Part model, mm, in its own coordinate system. A direction names the side the tool comes from. Round coordinates to 2 decimals unless told otherwise and drop trailing zeros. Write each loop counter-clockwise with the first axis right and the second up, starting at its lowest first coordinate (ties: lowest second). Pieces come first, ordered by that corner, then holes. Notation, with made-up numbers: (49, 0.25) -> (79, 0.25) arc R13 cw to (79, 11.25) -> close; hole circle Ø2 at (26, -11). An arc over 180 degrees is marked (long way). Use CSV: the item, a comma, the result in double quotes. Start each with the question number.
(1) Two-plate mould, pull along X, no slides. Class faces 1 (the flat face through (0, 12, 3.175)), 2 (the flat face through (-0.635, -9, 1)): released by +X, released by -X, zero draft, split by the parting line, or undercut.
(2) Which spindle directions (+Z, -Z, +X, -X, +Y, -Y) get a long thin tool onto all of the face, cutting with end or side? Do faces 3 (the flat face through (4.064, 0, 1)), 4 (the cylindrical face through (-4.556, -4.469, 1.436)), 5 (the cylindrical face through (10.37, -4.81, 1.89)), 6 (the cylindrical face through (8.496, -9.124, 1.61)). Say none if no direction does.
(3) Saw through at B-B (z = 1.15). Give the cut face in (x, y) (1 decimal).
(4) Saw through at A-A (x = 0). Give the cut face in (y, z) (3 decimals).
(5) Saw through at C-C (y = 1.25). Give the cut face in (x, z) (3 decimals).
(6) Saw through at D-D (x = -10.5). Give the cut face in (y, z) (3 decimals), plus the area to 4 significant figures.
(7) Drop flat-ended pins along their axis: pin 1 (1.3 mm diameter, centred on x = 8.5, z = 2, fed in from -Y); pin 2 (0.8 mm diameter, centred on y = 8.5, z = 1, fed in from -X); pin 3 (1.5 mm diameter, centred on x = -4, y = -5.5, fed in from -Z); pin 4 (5.5 mm diameter, centred on x = -4, y = -5, fed in from +Z). Give the stop position or say it passes through.
(8) Probe line 1 (X direction, y = 4, z = 2.2); line 2 (Y direction, x = 1.5, z = 1.05); line 3 (X direction, y = 5.5, z = 1.45). List the from-to ranges inside material, lowest first. Write a range as [from, to].
```python
from build123d import *

# Parameters (mm, degrees)
F0_W     = 8.128
F0_H     = 8.128
F1_DEPTH = 2.2606
F2_DEPTH = 0.635
F3_DEPTH = 3.175
F4_R     = 0.635


with BuildPart() as f1:
    # F0 (on Top) → F1 (new body)
    with BuildSketch(Plane.XY):
        with BuildLine():
            ThreePointArc((-6.3506963536, -0.635), (-4.5130128061, -4.5130128061), (-0.635, -6.3506963536))
            ThreePointArc((-0.635, -6.3506963536), (0, -6.3823639175), (0.635, -6.3506963536))
            ThreePointArc((0.635, -6.3506963536), (4.5130128061, -4.5130128061), (6.3506963536, -0.635))
            ThreePointArc((6.3506963536, -0.635), (6.3744421102, -0.3178945716), (6.3823639175, 0))
            ThreePointArc((6.3823639175, 0), (6.3744421102, 0.3178945716), (6.3506963536, 0.635))
            ThreePointArc((6.3506963536, 0.635), (4.5130128061, 4.5130128061), (0.635, 6.3506963536))
            ThreePointArc((0.635, 6.3506963536), (0, 6.3823639175), (-0.635, 6.3506963536))
            ThreePointArc((-0.635, 6.3506963536), (-4.5130128061, 4.5130128061), (-6.3506963536, 0.635))
            ThreePointArc((-6.3506963536, 0.635), (-6.3823639175, 0), (-6.3506963536, -0.635))
        make_face()
        Rectangle(F0_W, F0_H, mode=Mode.SUBTRACT)
        with BuildLine():
            Line((-0.635, -6.3506963536), (-0.635, -11.4123474798))
            ThreePointArc((-0.635, -11.4123474798), (0, -11.43), (0.635, -11.4123474798))
            Line((0.635, -11.4123474798), (0.635, -6.3506963536))
            ThreePointArc((0.635, -6.3506963536), (0, -6.3823639175), (-0.635, -6.3506963536))
        make_face()
        with BuildLine():
            ThreePointArc((0.635, 11.4123474798), (0, 11.43), (-0.635, 11.4123474798))
            Line((-0.635, 11.4123474798), (-0.635, 6.3506963536))
            ThreePointArc((-0.635, 6.3506963536), (0, 6.3823639175), (0.635, 6.3506963536))
            Line((0.635, 6.3506963536), (0.635, 11.4123474798))
        make_face()
        with BuildLine():
            Line((-8.8723474798, 0.635), (-8.8723474798, -0.635))
            Line((-8.8723474798, -0.635), (-6.3506963536, -0.635))
            ThreePointArc((-6.3506963536, -0.635), (-6.3823639175, 0), (-6.3506963536, 0.635))
            Line((-6.3506963536, 0.635), (-8.8723474798, 0.635))
        make_face()
        with BuildLine():
            Line((6.3506963536, -0.635), (8.8723474798, -0.635))
            Line((8.8723474798, -0.635), (8.8723474798, 0.635))
            Line((8.8723474798, 0.635), (6.3506963536, 0.635))
            ThreePointArc((6.3506963536, 0.635), (6.3744421102, 0.3178945716), (6.3823639175, 0))
            ThreePointArc((6.3823639175, 0), (6.3744421102, -0.3178945716), (6.3506963536, -0.635))
        make_face()
    extrude(amount=F1_DEPTH)

    # F0 (on Top) → F2 (join)
    with BuildSketch(Plane.XY):
        with BuildLine():
            ThreePointArc((-0.635, 11.4123474798), (-8.082230509, 8.082230509), (-11.4123474798, 0.635))
            Line((-11.4123474798, 0.635), (-8.8723474798, 0.635))
            Line((-8.8723474798, 0.635), (-6.3506963536, 0.635))
            ThreePointArc((-6.3506963536, 0.635), (-4.5130128061, 4.5130128061), (-0.635, 6.3506963536))
            Line((-0.635, 6.3506963536), (-0.635, 11.4123474798))
        make_face()
        with BuildLine():
            Line((8.8723474798, 0.635), (11.4123474798, 0.635))
            ThreePointArc((11.4123474798, 0.635), (8.082230509, 8.082230509), (0.635, 11.4123474798))
            Line((0.635, 11.4123474798), (0.635, 6.3506963536))
            ThreePointArc((0.635, 6.3506963536), (4.5130128061, 4.5130128061), (6.3506963536, 0.635))
            Line((6.3506963536, 0.635), (8.8723474798, 0.635))
        make_face()
        with BuildLine():
            ThreePointArc((0.635, -11.4123474798), (4.4682903074, -10.5204221269), (7.7718069116, -8.3811644375))
            ThreePointArc((7.7718069116, -8.3811644375), (10.3445014767, -4.8617064081), (11.4123474798, -0.635))
            Line((11.4123474798, -0.635), (8.8723474798, -0.635))
            Line((8.8723474798, -0.635), (6.3506963536, -0.635))
            ThreePointArc((6.3506963536, -0.635), (4.5130128061, -4.5130128061), (0.635, -6.3506963536))
            Line((0.635, -6.3506963536), (0.635, -11.4123474798))
        make_face()
        with BuildLine():
            ThreePointArc((-11.4123474798, -0.635), (-10.3445014767, -4.8617064081), (-7.7718069116, -8.3811644375))
            ThreePointArc((-7.7718069116, -8.3811644375), (-4.4682903074, -10.5204221269), (-0.635, -11.4123474798))
            Line((-0.635, -11.4123474798), (-0.635, -6.3506963536))
            ThreePointArc((-0.635, -6.3506963536), (-4.5130128061, -4.5130128061), (-6.3506963536, -0.635))
            Line((-6.3506963536, -0.635), (-8.8723474798, -0.635))
            Line((-8.8723474798, -0.635), (-11.4123474798, -0.635))
        make_face()
    extrude(amount=F2_DEPTH)

    # F0 (on Top) → F3 (join)
    with BuildSketch(Plane.XY):
        with BuildLine():
            ThreePointArc((-11.4123474798, 0.635), (-11.43, 0), (-11.4123474798, -0.635))
            Line((-11.4123474798, -0.635), (-8.8723474798, -0.635))
            Line((-8.8723474798, -0.635), (-8.8723474798, 0.635))
            Line((-8.8723474798, 0.635), (-11.4123474798, 0.635))
        make_face()
        with BuildLine():
            Line((8.8723474798, -0.635), (11.4123474798, -0.635))
            ThreePointArc((11.4123474798, -0.635), (11.4255860177, -0.317622658), (11.43, 0))
            ThreePointArc((11.43, 0), (11.4255860177, 0.317622658), (11.4123474798, 0.635))
            Line((11.4123474798, 0.635), (8.8723474798, 0.635))
            Line((8.8723474798, 0.635), (8.8723474798, -0.635))
        make_face()
        with BuildLine():
            ThreePointArc((8.4214084723, -9.5063073453), (11.581059701, -5.2123944786), (12.7, 0))
            ThreePointArc((12.7, 0), (-5.2123944786, 11.581059701), (-8.4214084723, -9.5063073453))
            Line((-8.4214084723, -9.5063073453), (-7.7718069116, -8.3811644375))
            ThreePointArc((-7.7718069116, -8.3811644375), (-10.3445014767, -4.8617064081), (-11.4123474798, -0.635))
            ThreePointArc((-11.4123474798, -0.635), (-11.43, 0), (-11.4123474798, 0.635))
            ThreePointArc((-11.4123474798, 0.635), (-8.082230509, 8.082230509), (-0.635, 11.4123474798))
            ThreePointArc((-0.635, 11.4123474798), (0, 11.43), (0.635, 11.4123474798))
            ThreePointArc((0.635, 11.4123474798), (8.082230509, 8.082230509), (11.4123474798, 0.635))
            ThreePointArc((11.4123474798, 0.635), (11.4255860177, 0.317622658), (11.43, 0))
            ThreePointArc((11.43, 0), (11.4255860177, -0.317622658), (11.4123474798, -0.635))
            ThreePointArc((11.4123474798, -0.635), (10.3445014767, -4.8617064081), (7.7718069116, -8.3811644375))
            Line((7.7718069116, -8.3811644375), (8.4214084723, -9.5063073453))
        make_face()
    extrude(amount=F3_DEPTH)

    # F4
    f4_edges = [f1.edges().sort_by_distance(p)[0] for p in [
        (-8.421408, -9.506307, 1.5875),
        (8.421408, -9.506307, 1.5875),
    ]]
    fillet(f4_edges, radius=F4_R)


solid = f1.part
```
Answers:
1,face 1,"zero draft"
1,face 2,"undercut"
2,face 3,"+Z, -Z"
2,face 4,"+Z, -Y"
2,face 5,"+Z"
2,face 6,"+Z, -Z, -Y"
3,outline,"(-11.4, -0.6) -> (-6.4, -0.6) arc R6.4 ccw to (-0.6, -6.4) -> (-0.6, -11.4) arc R11.4 ccw to (0.6, -11.4) -> (0.6, -6.4) arc R6.4 ccw to (6.4, -0.6) -> (11.4, -0.6) arc R11.4 cw to (7.8, -8.4) -> (8, -8.8) arc R0.6 ccw to (9, -8.9) arc R12.7 ccw (long way) to (-9, -8.9) arc R0.6 ccw to (-8, -8.8) -> (-7.8, -8.4) arc R11.4 cw to start; hole (-11.4, 0.6) -> (-6.4, 0.6) arc R6.4 cw to (-0.6, 6.4) -> (-0.6, 11.4) arc R11.4 ccw to start; hole (-4.1, -4.1) -> (4.1, -4.1) -> (4.1, 4.1) -> (-4.1, 4.1) -> close; hole (0.6, 6.4) arc R6.4 cw to (6.4, 0.6) -> (11.4, 0.6) arc R11.4 ccw to (0.6, 11.4) -> close"
4,outline,"(-11.43, 0) -> (-4.064, 0) -> (-4.064, 2.261) -> (-11.43, 2.261) -> close; (4.064, 0) -> (12.7, 0) -> (12.7, 3.175) -> (11.43, 3.175) -> (11.43, 2.261) -> (4.064, 2.261) -> close"
5,outline,"(-12.638, 0) -> (-4.064, 0) -> (-4.064, 2.261) -> (-6.259, 2.261) -> (-6.259, 0.635) -> (-11.361, 0.635) -> (-11.361, 3.175) -> (-12.638, 3.175) -> close; (4.064, 0) -> (12.638, 0) -> (12.638, 3.175) -> (11.361, 3.175) -> (11.361, 0.635) -> (6.259, 0.635) -> (6.259, 2.261) -> (4.064, 2.261) -> close"
6,outline,"(-7.144, 0) -> (7.144, 0) -> (7.144, 3.175) -> (4.516, 3.175) -> (4.516, 0.635) -> (0.635, 0.635) -> (0.635, 3.175) -> (-0.635, 3.175) -> (-0.635, 0.635) -> (-4.516, 0.635) -> (-4.516, 3.175) -> (-7.144, 3.175) -> close"
6,area,"25.65 mm²"
7,pin 1,"stops at y = -9.13"
7,pin 2,"stops at x = -9.78"
7,pin 3,"stops at z = 0"
7,pin 4,"stops at z = 2.26"
8,line 1,"x = [-12.05, -10.71], [-4.97, -4.06], [4.06, 4.97], [10.71, 12.05]"
8,line 2,"y = [-6.2, -4.06], [4.06, 6.2], [11.33, 12.61]"
8,line 3,"x = [-11.45, -10.02], [-3.24, 3.24], [10.02, 11.45]"
